from build123d import *

# Parameters (mm, degrees)
SKETCH_W             = 32
SKETCH_H             = 32
PAD_DEPTH            = 4
SKETCH001_W          = 32
SKETCH001_H          = 32
SKETCH001_R          = 1
PAD001_DEPTH         = 9.5
SKETCH002_W          = 30
SKETCH002_H          = 30
POCKET_DEPTH         = 3.5
SKETCH003_W          = 1
SKETCH003_H          = 17.8
POCKET001_DEPTH      = 6.5
SKETCH004_R          = 1
POCKET002_DEPTH      = 4.001
POCKET002_DEPTH_BACK = 9.501
POCKET003_DEPTH      = 3


with BuildPart() as part:
    # Sketch → Pad (new body)
    with BuildSketch(Plane.XZ):
        with Locations((0, 16)):
            Rectangle(SKETCH_W, SKETCH_H)
    extrude(amount=PAD_DEPTH)

    # Sketch001 (on Face6 of Pad) → Pad001 (join)
    with BuildSketch(Plane.XZ.offset(4)):
        with Locations((0, 16)):
            Rectangle(SKETCH001_W, SKETCH001_H)
        with Locations((-11.25, 4.75)):
            Circle(SKETCH001_R, mode=Mode.SUBTRACT)
        with Locations((11.25, 4.75)):
            Circle(SKETCH001_R, mode=Mode.SUBTRACT)
        with Locations((11.25, 27.25)):
            Circle(SKETCH001_R, mode=Mode.SUBTRACT)
        with Locations((-11.25, 27.25)):
            Circle(SKETCH001_R, mode=Mode.SUBTRACT)
        with BuildLine():
            Line((-15, 24.9), (-11.4, 24.9))
            ThreePointArc((-11.4, 24.9), (-9.632233, 25.632233), (-8.9, 27.4))
            Line((-8.9, 27.4), (-8.9, 31))
            Line((-8.9, 31), (8.9, 31))
            Line((8.9, 31), (8.9, 27.4))
            ThreePointArc((8.9, 27.4), (9.632233, 25.632233), (11.4, 24.9))
            Line((11.4, 24.9), (15, 24.9))
            Line((15, 24.9), (15, 7.1))
            Line((11.4, 7.1), (15, 7.1))
            ThreePointArc((11.4, 7.1), (9.632233, 6.367767), (8.9, 4.6))
            Line((8.9, 1), (8.9, 4.6))
            Line((8.9, 1), (-8.9, 1))
            Line((-8.9, 4.6), (-8.9, 1))
            ThreePointArc((-8.9, 4.6), (-9.632233, 6.367767), (-11.4, 7.1))
            Line((-15, 7.1), (-11.4, 7.1))
            Line((-15, 7.1), (-15, 24.9))
        make_face(mode=Mode.SUBTRACT)
    extrude(amount=PAD001_DEPTH)

    # Sketch002 (on Face9 of Pad001) → Pocket (cut)
    with BuildSketch(Plane.XZ.offset(13.5)):
        with Locations((0, 16)):
            Rectangle(SKETCH002_W, SKETCH002_H)
    extrude(amount=-POCKET_DEPTH, mode=Mode.SUBTRACT)

    # Sketch003 (on Face9 of Pocket) → Pocket001 (cut)
    with BuildSketch(Plane.XZ.offset(13.5)):
        with Locations((15.5, 16)):
            Rectangle(SKETCH003_W, SKETCH003_H)
    extrude(amount=-POCKET001_DEPTH, mode=Mode.SUBTRACT)

    # Sketch004 (on Face35 of Pocket001) → Pocket002 (cut, two sides)
    with BuildSketch(Plane.XZ.offset(4)) as pocket002_sk:
        with Locations((-11.25, 27.25)):
            Circle(SKETCH004_R)
        with Locations((11.25, 27.25)):
            Circle(SKETCH004_R)
        with Locations((11.25, 4.75)):
            Circle(SKETCH004_R)
        with Locations((-11.25, 4.75)):
            Circle(SKETCH004_R)
    extrude(amount=-POCKET002_DEPTH, mode=Mode.SUBTRACT)
    extrude(pocket002_sk.sketch, amount=POCKET002_DEPTH_BACK, mode=Mode.SUBTRACT)

    # Sketch005 (on Face4 of Pocket002) → Pocket003 (cut)
    with BuildSketch(Plane(origin=(0, 0, 0), x_dir=(1, 0, 0), z_dir=(0, 1, 0))):
        Polygon((-10.125, -6.698557), (-9, -4.75), (-10.125, -2.801443), (-12.375, -2.801443), (-13.5, -4.75), (-12.375, -6.698557), align=None)
        Polygon((12.375, -6.698557), (13.5, -4.75), (12.375, -2.801443), (10.125, -2.801443), (9, -4.75), (10.125, -6.698557), align=None)
        Polygon((12.375, -29.198557), (13.5, -27.25), (12.375, -25.301443), (10.125, -25.301443), (9, -27.25), (10.125, -29.198557), align=None)
        Polygon((-10.125, -29.198557), (-9, -27.25), (-10.125, -25.301443), (-12.375, -25.301443), (-13.5, -27.25), (-12.375, -29.198557), align=None)
    extrude(amount=-POCKET003_DEPTH, mode=Mode.SUBTRACT)


solid = part.part
CAD build for the part. Positions are in the model's coordinates, mm. A direction names the side the tool comes from. Coordinates: 2 decimals unless noted, no trailing zeros. Write each loop counter-clockwise with the first axis right and the second up, starting at its lowest first coordinate (ties: lowest second). Pieces come first, ordered by that corner, then holes. Notation, with made-up numbers: (14.5, -10.75) - (50.5, -10.75) arc R7 ccw to (50.5, -0.75) - close; hole circle Ø3 at (27.5, 35). An arc over 180 degrees is marked (long way). Use a Markdown table: item, result. Add a question column.
Item 1: Band-saw the part on D-D, the plane y = -11.75. Give the cut face in (x, z), and give its area (3 significant figures).
Item 2: Band-saw the part on B-B, the plane z = 12.5. Give the cut face in (x, y).
Item 3: Band-saw the part on C-C, the plane y = -5.5. Give the cut face in (x, z).
Item 4: 3-axis set-ups, long thin cutter, end or side, ignore diameter. For faces 1 (the face through (11, -1, 6.699)), 2 (the face through (8.9, -7, 29)): which of +Z, -Z, +X, -X, +Y, -Y reach the whole face in a straight line?
Item 5: Drill centre lines: L1, parallel to X at y = -7.25, z = 27.25; L2, parallel to Z at x = -11.25, y = -7.75; L3, parallel to X at y = -11.75, z = 27. Where is each one in solid material? Low to high. Write a range as from..to.
Item 6: Flat gauge pins, fed straight in: pin 1 (1.5 mm diameter, centred on x = 0.5, z = 13, fed in from -Y); pin 2 (1.1 mm diameter, centred on x = 15.5, z = 19.5, fed in from -Y). Where does each tip first touch, or does it go through?
Item 7: Band-saw the part on A-A, the plane y = -0.75. Give the cut face in (x, z) (3 decimals), and give its area (3 significant figures).
Numbers:
| question | item | result |
|---|---|---|
| 1 | outline | (-16, 0) - (16, 0) - (16, 7.1) - (15, 7.1) - (15, 1) - (-15, 1) - (-15, 31) - (15, 31) - (15, 24.9) - (16, 24.9) - (16, 32) - (-16, 32) - close |
| 1 | area | 106 mm2 |
| 2 | outline | (-16, -13.5) - (-15, -13.5) - (-15, -4) - (15, -4) - (15, -7) - (16, -7) - (16, 0) - (-16, 0) - close |
| 3 | outline | (-16, 0) - (16, 0) - (16, 32) - (-16, 32) - close; hole (-15, 7.1) - (-11.4, 7.1) arc R2.5 cw to (-8.9, 4.6) - (-8.9, 1) - (8.9, 1) - (8.9, 4.6) arc R2.5 cw to (11.4, 7.1) - (15, 7.1) - (15, 24.9) - (11.4, 24.9) arc R2.5 cw to (8.9, 27.4) - (8.9, 31) - (-8.9, 31) - (-8.9, 27.4) arc R2.5 cw to (-11.4, 24.9) - (-15, 24.9) - close; hole circle Ø2 at (-11.25, 4.75); hole circle Ø2 at (-11.25, 27.25); hole circle Ø2 at (11.25, 4.75); hole circle Ø2 at (11.25, 27.25) |
| 4 | face 1 | +Y |
| 4 | face 2 | -Y |
| 5 | L1 | -16..-12.25, -10.25..-8.9, 8.9..10.25, 12.25..16 |
| 5 | L2 | 0..3.75, 5.75..7.1, 24.9..26.25, 28.25..32 |
| 5 | L3 | -16..-15, 15..16 |
| 6 | pin 1 | y = -4 |
| 6 | pin 2 | y = -7 |
| 7 | outline | (-16, 0) - (16, 0) - (16, 32) - (-16, 32) - close; hole (-13.5, 4.75) - (-12.375, 2.801) - (-10.125, 2.801) - (-9, 4.75) - (-10.125, 6.699) - (-12.375, 6.699) - close; hole (-13.5, 27.25) - (-12.375, 25.301) - (-10.125, 25.301) - (-9, 27.25) - (-10.125, 29.199) - (-12.375, 29.199) - close; hole (9, 4.75) - (10.125, 2.801) - (12.375, 2.801) - (13.5, 4.75) - (12.375, 6.699) - (10.125, 6.699) - close; hole (9, 27.25) - (10.125, 25.301) - (12.375, 25.301) - (13.5, 27.25) - (12.375, 29.199) - (10.125, 29.199) - close |
| 7 | area | 971 mm2 |
